Can you work these out from the model? Positions are in its coordinate system, mm. Round coordinates to 2 decimals unless told otherwise and drop trailing zeros. Loops run counter-clockwise (first coordinate to the right, second up) from the corner with the lowest first, then second, coordinate; pieces in that order, holes last. Notation, with made-up numbers: (74.5, -9) -> (112.5, -9) arc R22 ccw to (112.5, 0) -> close; hole circle Ø7 at (8.25, -7.5). An arc over 180 degrees is marked (long way). Use a Markdown table: item, result.
from build123d import *

# Parameters (mm, degrees)
SKETCH_1_R               = 48.5
SKETCH_1_R_2             = 32
EXTRUDE_1_DEPTH          = 4
SKETCH_2_R               = 3
CUT_EXTRUDE_1_DEPTH      = 18.6
PATTERN_CIRCULAR_1_COUNT = 12


with BuildPart() as part:
    # Эскиз1 → Бобышка-Вытянуть1 (new body)
    with BuildSketch(Plane.XY):
        Circle(SKETCH_1_R)
        Circle(SKETCH_1_R_2, mode=Mode.SUBTRACT)
    extrude(amount=EXTRUDE_1_DEPTH)

    # Эскиз2 → Вырез-Вытянуть1 (cut)
    with BuildSketch(Plane(origin=(0, 0, 0), x_dir=(-1, 0, 0), z_dir=(0, 0, -1))):
        with Locations((0, 40)):
            Circle(SKETCH_2_R)
    cut_extrude_1 = extrude(amount=-CUT_EXTRUDE_1_DEPTH, mode=Mode.SUBTRACT)

    # Круговой массив1: Вырез-Вытянуть1 ×12 about axis
    pattern_circular_1_axis = Axis((0, 0, 0), (0, 0, 1))
    for i in range(1, PATTERN_CIRCULAR_1_COUNT):
        add(cut_extrude_1.rotate(pattern_circular_1_axis, i * 360 / PATTERN_CIRCULAR_1_COUNT), mode=Mode.SUBTRACT)


solid = part.part
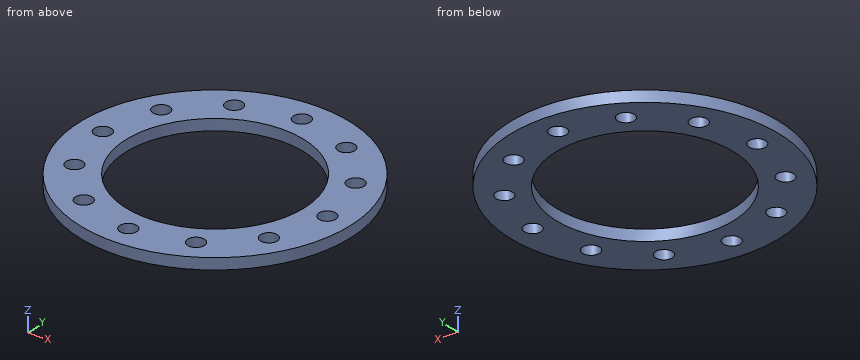
1. I want a section at A-A (x = -7.5). Please give me the cut outline in (y, z).
Answer sheet:
| item | result |
|---|---|
| outline | (-47.92, 0) -> (-31.11, 0) -> (-31.11, 4) -> (-47.92, 4) -> close; (31.11, 0) -> (47.92, 0) -> (47.92, 4) -> (31.11, 4) -> close |
2. I need wall thicknesses on line 1 (Y direction, x = 0, z = 1.4); line 2 (X direction, y = -33, z = 3.15); line 3 (Y direction, x = -34.5, z = 1.2). Which ranges of each line are inside material? Lowest first, please.
Answer sheet:
| item | result |
|---|---|
| line 1 | y = -48.5 to -43, -37 to -32, 32 to 37, 43 to 48.5 |
| line 2 | x = -35.54 to -22.51, -17.49 to 17.49, 22.51 to 35.54 |
| line 3 | y = -34.09 to -23, -17 to 17, 23 to 34.09 |
3. I want a section at D-D (x = 20). Please give me the cut outline in (y, z), plus the area to 3 significant figures.
Answer sheet:
| item | result |
|---|---|
| outline | (-44.18, 0) -> (-37.64, 0) -> (-37.64, 4) -> (-44.18, 4) -> close; (-31.64, 0) -> (-24.98, 0) -> (-24.98, 4) -> (-31.64, 4) -> close; (24.98, 0) -> (31.64, 0) -> (31.64, 4) -> (24.98, 4) -> close; (37.64, 0) -> (44.18, 0) -> (44.18, 4) -> (37.64, 4) -> close |
| area | 106 mm² |
4. I want a section at B-B (y = -15.5). Please give me the cut outline in (x, z), plus the area to 3 significant figures.
Answer sheet:
| item | result |
|---|---|
| outline | (-45.96, 0) -> (-28, 0) -> (-28, 4) -> (-45.96, 4) -> close; (28, 0) -> (45.96, 0) -> (45.96, 4) -> (28, 4) -> close |
| area | 144 mm² |
5. Will these pins go through, and if not, where does the flat tip stop? pin 1 Ø5 at (x, y) = (0, 40) entering from +Z; pin 2 Ø1.5 at (y, z) = (6, 1) entering from +X (3 decimals).
Answer sheet:
| item | result |
|---|---|
| pin 1 | passes through |
| pin 2 | stops at x = 48.215 |
6. I want a section at C-C (y = -35). Please give me the cut outline in (x, z), plus the area to 3 significant figures.
Answer sheet:
| item | result |
|---|---|
| outline | (-33.57, 0) -> (-22.98, 0) -> (-22.98, 4) -> (-33.57, 4) -> close; (-17.02, 0) -> (17.02, 0) -> (17.02, 4) -> (-17.02, 4) -> close; (22.98, 0) -> (33.57, 0) -> (33.57, 4) -> (22.98, 4) -> close |
| area | 221 mm² |
